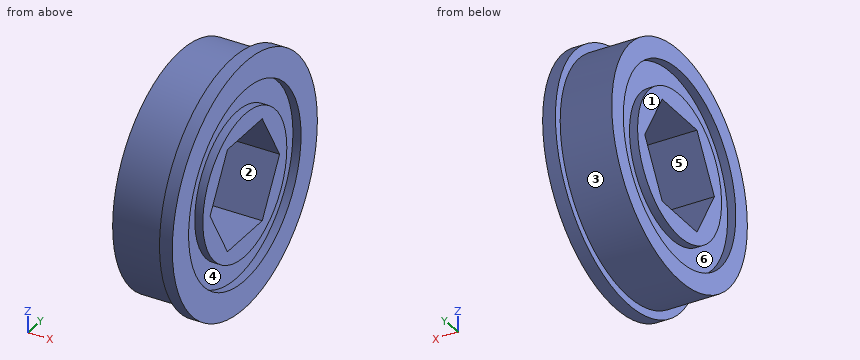
Autodesk Inventor part; units mm, degrees
ref_plane "YZ Plane" through (0, 0, 0) normal (1, 0, 0) x (0, 1, 0)
ref_plane "XZ Plane" through (0, 0, 0) normal (0, 1, 0) x (-1, 0, 0)
ref_plane "XY Plane" through (0, 0, 0) normal (0, 0, 1) x (1, 0, 0)
sketch "Sketch1" plane through (0, 0, 0) normal (0, 0, 1) x (1, 0, 0)
  line L0 (0, 14.2875) -> (6.35, 14.2875)
  line L1 (6.35, 14.2875) -> (6.35, 15.2875)
  line L2 (6.35, 15.2875) -> (7.9248, 15.2875)
  line L3 (7.9248, 15.2875) -> (7.9248, 6.35)
  line L4 (7.9248, 6.35) -> (0, 6.35)
  line L5 (0, 6.35) -> (0, 14.2875)
  line L6 (0, 0) -> (7.9248, 0)
  line L7 (0, 11.85) -> (1, 11.85)
  line L8 (1, 11.85) -> (1, 8.85)
  line L9 (1, 8.85) -> (0, 8.85)
  line L10 (0, 8.85) -> (0, 11.85)
  line L11 (7.9248, 8.85) -> (6.9248, 8.85)
  line L12 (6.9248, 8.85) -> (6.9248, 11.85)
  line L13 (6.9248, 11.85) -> (7.9248, 11.85)
  line L14 (7.9248, 11.85) -> (7.9248, 8.85)
  dimension "d0" = 7.9248
  dimension "d2" = 12.7
  dimension "d3" = 28.575
  dimension "d4" = 1.5748
  dimension "d5" = 1
  dimension "d7" = 1
  dimension "d8" = 3
  dimension "d9" = 2.5
revolve "Revolution1" add sketch "Sketch1" angle 360 about axis through (0, 0, 0) along (1, 0, 0) contours L0 L1 L2 L3 L13 L12 L11 L4 L5 L9 L8 L7
sketch "Sketch2" plane through (7.9248, 0, 0) normal (1, 0, 0) x (0, 0, -1)
  circle A0 centre (0, 0) radius 8.85
  circle A1 centre (0, 0) radius 6.35
  line L0 (0, 7.3323) -> (6.35, 3.6662)
  line L1 (6.35, 3.6662) -> (6.35, -3.6662)
  line L2 (6.35, -3.6662) -> (0, -7.3323)
  line L3 (0, -7.3323) -> (-6.35, -3.6662)
  line L4 (-6.35, -3.6662) -> (-6.35, 3.6662)
  line L5 (-6.35, 3.6662) -> (0, 7.3323)
extrude "Extrusion1" cut sketch "Sketch2" against normal through all contours L1 L2 A1 | A1 L0 L1 | A1 L5 L0 | L2 L3 A1 | A1 L4 L5 | L3 L4 A1
properties part number "RoundBearing-1-2-inch"
The listing builds one solid part. Answer for the finished solid, in the listing's coordinates (mm). Face numbers are marked on the shaded views. A direction names the side the tool comes from. Coordinates: 2 decimals unless noted, no trailing zeros. Loops run counter-clockwise (first coordinate to the right, second up) from the corner with the lowest first, then second, coordinate; pieces in that order, holes last. Notation, with made-up numbers: M 75.5,63 L 132.5,63 A15 cw 132.5,69 Z; hole C 42,81 d11. An arc over 180 degrees is marked long. Answer as a JSON object with one key per item and string values. Group by question number.
Item 1: Determine the mould class of the marked faces 1, 2 and 3 for opening direction Z: +Z half, -Z half, draft (parallel to the pull), parting line (faces both ways), or undercut.
Item 2: Consider L1, parallel to Z at x = 0.7, y = 0; L2, parallel to Z at x = 0.5, y = -6; L3, parallel to Z at x = 3.5, y = -7. Determine where each line is inside the solid, lowest interval first.
Item 3: Section A-A (y = 0) is taken. Write down the section's boundary in (x, z).
Item 4: Section D-D (z = -7) is taken. Write down the section's boundary in (x, y).
Item 5: Each of these flat-tipped pins is pushed along its axis until it touches: P1, Ø1, axis at x = 3, z = -2, coming from the +Y side; P2, Ø1, axis at x = 1.5, z = -5.5, coming from the +Y side; P3, Ø1, axis at x = 5, z = 11, coming from the -Y side. Where does it stop, or does it pass through?
Item 6: Section C-C (z = -1.5) is taken. Write down the section's boundary in (x, y), and give its area (3 significant figures).
Item 7: Which of the six approach directions +Z, -Z, +X, -X, +Y, -Y give full straight-line access (tool end or side, diameter ignored) to the marked faces 4, 5 and 6?
Solved:
{
 "1": {"face 1": "draft", "face 2": "undercut", "face 3": "parting line"},
 "2": {"L1": "z = -14.29 to -11.85, -8.85 to -6.35, 6.35 to 8.85, 11.85 to 14.29", "L2": "z = -12.97 to -10.22, -6.51 to -2.31, 2.31 to 6.51, 10.22 to 12.97", "L3": "z = -12.46 to -0.58, 0.58 to 12.46"},
 "3": {"outline": "M 0,-14.29 L 6.35,-14.29 L 6.35,-15.29 L 7.92,-15.29 L 7.92,-11.85 L 6.92,-11.85 L 6.92,-8.85 L 7.92,-8.85 L 7.92,-6.35 L 0,-6.35 L 0,-8.85 L 1,-8.85 L 1,-11.85 L 0,-11.85 Z; M 0,6.35 L 7.92,6.35 L 7.92,8.85 L 6.92,8.85 L 6.92,11.85 L 7.92,11.85 L 7.92,15.29 L 6.35,15.29 L 6.35,14.29 L 0,14.29 L 0,11.85 L 1,11.85 L 1,8.85 L 0,8.85 Z"},
 "4": {"outline": "M 0,-12.46 L 6.35,-12.46 L 6.35,-13.59 L 7.92,-13.59 L 7.92,-9.56 L 6.92,-9.56 L 6.92,-5.42 L 7.92,-5.42 L 7.92,5.42 L 6.92,5.42 L 6.92,9.56 L 7.92,9.56 L 7.92,13.59 L 6.35,13.59 L 6.35,12.46 L 0,12.46 L 0,9.56 L 1,9.56 L 1,5.42 L 0,5.42 L 0,-5.42 L 1,-5.42 L 1,-9.56 L 0,-9.56 Z"},
 "5": {"P1": "stops at y = 14.21", "P2": "stops at y = 13.38", "P3": "stops at y = -9.69"},
 "6": {"outline": "M 0,-14.21 L 6.35,-14.21 L 6.35,-15.21 L 7.92,-15.21 L 7.92,-11.75 L 6.92,-11.75 L 6.92,-8.72 L 7.92,-8.72 L 7.92,-6.47 L 0,-6.47 L 0,-8.72 L 1,-8.72 L 1,-11.75 L 0,-11.75 Z; M 0,6.47 L 7.92,6.47 L 7.92,8.72 L 6.92,8.72 L 6.92,11.75 L 7.92,11.75 L 7.92,15.21 L 6.35,15.21 L 6.35,14.21 L 0,14.21 L 0,11.75 L 1,11.75 L 1,8.72 L 0,8.72 Z", "area": "114 mm2"},
 "7": {"face 4": "+X", "face 5": "+X, -X", "face 6": "-X"}
}
